Geometry check sheet. Reference: the model listing, model coordinates, mm. A direction names the side the tool comes from. Coordinates: 2 decimals unless noted, no trailing zeros. Loops run counter-clockwise (first coordinate to the right, second up) from the corner with the lowest first, then second, coordinate; pieces in that order, holes last. Notation, with made-up numbers: (45, 40.25) - (92, 40.25) arc R18 cw to (92, 53.25) - close; hole circle Ø7 at (-6.75, -32). An arc over 180 degrees is marked (long way). One line per item, written item: value.
from build123d import *

# Parameters (mm, degrees)
M5_CLEARANCE_HOLE1_D           = 5.5
M5_CLEARANCE_HOLE1_CSINK_D     = 12
M5_CLEARANCE_HOLE1_CSINK_ANGLE = 90


with BuildPart() as part:
    # Sketch1 → Revolve1 (revolve)
    with BuildSketch(Plane.XY):
        Polygon((-45, 0), (-16, 0), (-16, -13), (-10, -13), (-10, -62), (-16, -62), (-16, -75), (-27.5, -75), (-27.5, -12), (-45, -12), align=None)
    revolve(axis=Axis((0, 0, 0), (0, 1, 0)))

    # M5 Clearance Hole1 (through all)
    with Locations(Plane(origin=(0, -12, 0), x_dir=(-1, 0, 0), z_dir=(0, -1, 0))):
        with Locations((-35.5, 0), (0, -35.5), (35.5, 0), (0, 35.5)):
            CounterSinkHole(M5_CLEARANCE_HOLE1_D / 2, M5_CLEARANCE_HOLE1_CSINK_D / 2, counter_sink_angle=M5_CLEARANCE_HOLE1_CSINK_ANGLE)


solid = part.part
(1) Cross-section at D-D on y = -70. Record the cut outline in (x, z), and give its area (3 significant figures).
Reply:
outline: circle Ø55 at (0, 0); hole circle Ø32 at (0, 0)
area: 1,570 mm2
(2) Material ranges on probe 1 along Z at (x, y) = (0, -7); probe 2 along Z at (x, y) = (0, -71); probe 3 along Z at (x, y) = (2, -8), recorded low to high. Write a range as from..to.
Reply:
probe 1: -45..-38.25, -32.75..-16, 16..32.75, 38.25..45
probe 2: -27.5..-16, 16..27.5
probe 3: -44.96..-37.39, -33.61..-15.87, 15.87..33.61, 37.39..44.96
(3) Release check for a two-part mould opening along X. For faces 4 (the face through (12, -75, -12)), 5 (the face through (-32.726, -8.908, -0.873)), 6 (the face through (0.2, -13, -10.4)), 7 (the face through (-20.765, -5.916, -39.923)) record: pulls with the +X half, pulls with the -X half, needs draft (parallel to the pull), parting line crosses it, or undercut.
Reply:
face 4: needs draft
face 5: undercut
face 6: undercut
face 7: parting line crosses it
(4) Cross-section at A-A on x = 0. State how many separate pieces and enclosed holes the cut face has, and give its area (3 significant figures).
Reply:
separate pieces: 4
enclosed holes: 0
area: 2,580 mm2
(5) Go/stop test with flat-tipped pins: pin 1 Ø6 at (y, z) = (-53, 28.5) entering from -X; pin 2 Ø1 at (y, z) = (-32, 14) entering from -X; pin 3 Ø7 at (x, z) = (0, 35.5) entering from -Y. Record where each tip stops, or that it passes through.
Reply:
pin 1: x = -10.3
pin 2: x = -23.96
pin 3: y = -9.5
(6) Cross-section at C-C on x = 35.5. Record the cut outline in (y, z), and give its area (3 significant figures).
Reply:
outline: (-12, -27.65) - (0, -27.65) - (0, -2.75) - (-8.75, -2.75) - (-12, -6) - close; (-12, 6) - (-8.75, 2.75) - (0, 2.75) - (0, 27.65) - (-12, 27.65) - close
area: 587 mm2
(7) Access from +Z, -Z, +X, -X, +Y, -Y to the whole of each face (thin tool, end or side, straight path). Record for faces 1 (the face through (1, 0, -19)), 2 (the face through (3.47, -6.59, -15.62)), 3 (the face through (-0.2, -62, -10.4)).
Reply:
face 1: +Z, -Z, +X, -X, +Y
face 2: +Y
face 3: -Y
(8) Cross-section at B-B on z = 35.5. Record the cut outline in (x, y), and give its area (3 significant figures).
Reply:
outline: (-27.65, -12) - (-6, -12) - (-2.75, -8.75) - (-2.75, 0) - (-27.65, 0) - close; (2.75, -8.75) - (6, -12) - (27.65, -12) - (27.65, 0) - (2.75, 0) - close
area: 587 mm2
